Geometry check sheet. Reference: the model listing, model coordinates, mm. A direction names the side the tool comes from. Coordinates: 2 decimals unless noted, no trailing zeros. Loops run counter-clockwise (first coordinate to the right, second up) from the corner with the lowest first, then second, coordinate; pieces in that order, holes last.
from build123d import *

# Parameters (mm, degrees)
SKETCH1_R           = 7.9375
SKETCH1_R_2         = 2.0955
WHOLE_PART_DEPTH    = 6.35
SKETCH2_R           = 8.89
BEARING_DEPTH_DEPTH = 1.016
NUT_POCKET_DEPTH    = 3.96875


with BuildPart() as part:
    # Sketch1 → whole-part (new body)
    with BuildSketch(Plane(origin=(0, 0, 0), x_dir=(1, 0, 0), z_dir=(0, 1, 0))):
        with BuildLine():
            Line((-21.166666667, 5.986837414), (-4.233333333, 11.973674828))
            ThreePointArc((-4.233333333, 11.973674828), (0, 12.7), (4.233333333, 11.973674828))
            Line((4.233333333, 11.973674828), (21.166666667, 5.986837414))
            ThreePointArc((21.166666667, 5.986837414), (25.4, 0), (21.166666667, -5.986837414))
            Line((21.166666667, -5.986837414), (4.233333333, -11.973674828))
            ThreePointArc((4.233333333, -11.973674828), (0, -12.7), (-4.233333333, -11.973674828))
            Line((-4.233333333, -11.973674828), (-21.166666667, -5.986837414))
            ThreePointArc((-21.166666667, -5.986837414), (-25.4, 0), (-21.166666667, 5.986837414))
        make_face()
        with Locations(Location((0, 0, 0), (0, 0, 270))):
            Circle(SKETCH1_R, mode=Mode.SUBTRACT)
        with Locations(Location((-19.05, 0, 0), (0, 0, 270))):
            Circle(SKETCH1_R_2, mode=Mode.SUBTRACT)
        with Locations(Location((19.05, 0, 0), (0, 0, 270))):
            Circle(SKETCH1_R_2, mode=Mode.SUBTRACT)
    extrude(amount=WHOLE_PART_DEPTH)

    # Sketch2 → bearing-depth (cut)
    with BuildSketch(Plane(origin=(0, 0, 0), x_dir=(-1, 0, 0), z_dir=(0, -1, 0))):
        with Locations(Location((0, 0, 0), (0, 0, 90))):
            Circle(SKETCH2_R)
    extrude(amount=-BEARING_DEPTH_DEPTH, mode=Mode.SUBTRACT)

    # Sketch3 → nut-pocket (cut)
    with BuildSketch(Plane(origin=(0, 6.35, 0), x_dir=(1, 0, 0), z_dir=(0, 1, 0))):
        Polygon((-23.415625, 2.520494769), (-23.415625, -2.520494769), (-19.05, -5.040989538), (-14.684375, -2.520494769), (-14.684375, 2.520494769), (-19.05, 5.040989538), align=None)
        Polygon((19.05, 5.040989538), (14.684375, 2.520494769), (14.684375, -2.520494769), (19.05, -5.040989538), (23.415625, -2.520494769), (23.415625, 2.520494769), align=None)
    extrude(amount=-NUT_POCKET_DEPTH, mode=Mode.SUBTRACT)


solid = part.part
(1) Access from +Z, -Z, +X, -X, +Y, -Y to the whole of each face (thin tool, end or side, straight path). Record for faces 1 (the cylindrical face through (-8.68, 0.5, 1.93)), 2 (the flat face through (16.9, 4.4, -3.8)), 3 (the cylindrical face through (-16.97, 1.17, -0.27)).
Findings:
face 1: -Y
face 2: +Y
face 3: +Y, -Y
(2) Sectioned sample at B-B on z = 0. Record the cut outline in (x, y).
Findings:
outline: (-25.4, 0) - (-21.15, 0) - (-21.15, 2.38) - (-23.42, 2.38) - (-23.42, 6.35) - (-25.4, 6.35) - close; (-16.95, 0) - (-8.89, 0) - (-8.89, 1.02) - (-7.94, 1.02) - (-7.94, 6.35) - (-14.68, 6.35) - (-14.68, 2.38) - (-16.95, 2.38) - close; (7.94, 1.02) - (8.89, 1.02) - (8.89, 0) - (16.95, 0) - (16.95, 2.38) - (14.68, 2.38) - (14.68, 6.35) - (7.94, 6.35) - close; (21.15, 0) - (25.4, 0) - (25.4, 6.35) - (23.42, 6.35) - (23.42, 2.38) - (21.15, 2.38) - close
(3) Scan lines: L1, parallel to X at y = 2.3, z = 0; L2, parallel to X at y = 0.25, z = 0; L3, parallel to Z at x = 0, y = 3.2. Record each from-to range of solid material in increasing order.
Findings:
L1: x = -25.4 to -21.15, -16.95 to -7.94, 7.94 to 16.95, 21.15 to 25.4
L2: x = -25.4 to -21.15, -16.95 to -8.89, 8.89 to 16.95, 21.15 to 25.4
L3: z = -12.7 to -7.94, 7.94 to 12.7
(4) Draft check along X on faces 4 (the flat face through (12.819, 3.131, 8.938)), 5 (the flat face through (-12.581, 3.131, 9.022)), 6 (the flat face through (17, 2.381, 1)), 7 (the flat face through (-5, 0, 8)). Enter one of: +X half, -X half, draft (parallel to the pull), parting line (faces both ways), or undercut.
Findings:
face 4: +X half
face 5: -X half
face 6: undercut
face 7: draft
(5) Sectioned sample at C-C on x = 0. Record the cut outline in (y, z), and give its area (3 significant figures).
Findings:
outline: (0, -12.7) - (6.35, -12.7) - (6.35, -7.94) - (1.02, -7.94) - (1.02, -8.89) - (0, -8.89) - close; (0, 8.89) - (1.02, 8.89) - (1.02, 7.94) - (6.35, 7.94) - (6.35, 12.7) - (0, 12.7) - close
area: 58.5 mm2
(6) Sectioned sample at A-A on y = 3. State how many separate pieces and enclosed holes the cut face has, and give its area (3 significant figures).
Findings:
separate pieces: 1
enclosed holes: 3
area: 563 mm2
(7) Sectioned sample at D-D on z = 3.5. Record the cut outline in (x, y), and give its area (3 significant figures).
Findings:
outline: (-24.35, 0) - (-8.17, 0) - (-8.17, 1.02) - (-7.12, 1.02) - (-7.12, 6.35) - (-16.38, 6.35) - (-16.38, 2.38) - (-21.72, 2.38) - (-21.72, 6.35) - (-24.35, 6.35) - close; (7.12, 1.02) - (8.17, 1.02) - (8.17, 0) - (24.35, 0) - (24.35, 6.35) - (21.72, 6.35) - (21.72, 2.38) - (16.38, 2.38) - (16.38, 6.35) - (7.12, 6.35) - close
area: 174 mm2
(8) Gauge pin test, flat ends, axial feed: pin 1 Ø1.5 at (y, z) = (2.5, 1.5) entering from +X; pin 2 Ø1.5 at (x, y) = (9, 2) entering from +Z; pin 3 Ø5.5 at (x, z) = (19.05, 0) entering from +Y. Record the tip position at first contact, or that the pin passes through.
Findings:
pin 1: stops at x = 25.36
pin 2: stops at z = 10.55
pin 3: stops at y = 2.38
